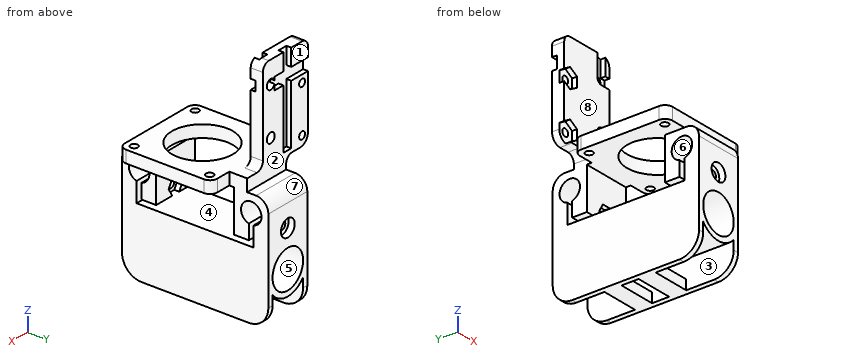
```python
from build123d import *

# Parameters (mm, degrees)
SKETCH_1_W                = 15.5
SKETCH_1_H                = 11.302783866
EXTRUDE_1_DEPTH           = 60
SKETCH_2_R                = 4.2
CUT_EXTRUDE_1_DEPTH       = 90
CUT_EXTRUDE_2_DEPTH       = 40
SKETCH_4_W                = 15.5
SKETCH_4_H                = 19.5
SKETCH_4_H_2              = 7
CUT_EXTRUDE_3_DEPTH       = 6
FILLET_1_R                = 5
FILLET_2_R                = 8
SKETCH_13_R               = 1.8
CUT_EXTRUDE_9_DEPTH       = 75
SKETCH_8_W                = 19.8
SKETCH_8_H                = 7.315078523
SKETCH_8_H_2              = 8
EXTRUDE_3_DEPTH           = 5
SKETCH_10_R               = 12.5
SKETCH_10_R_2             = 1.5
CUT_EXTRUDE_6_DEPTH       = 5
FILLET_4_R                = 3
CUT_EXTRUDE_10_DEPTH      = 34
CUT_EXTRUDE_10_DEPTH_BACK = 2
SKETCH_15_R               = 3.5
CUT_EXTRUDE_11_DEPTH      = 2.5
CUT_EXTRUDE_START         = -2.5
SKETCH_16_R               = 3.5
CUT_EXTRUDE_12_DEPTH      = 2.5
SKETCH_17_W               = 22.9
SKETCH_17_H               = 5
EXTRUDE_4_DEPTH           = 38
SKETCH_18_R               = 1.5
SKETCH_18_R_2             = 2
CUT_EXTRUDE_13_DEPTH      = 36.5
CUT_EXTRUDE_14_DEPTH      = 2
FILLET_5_R                = 3
SKETCH_20_W               = 4.5
SKETCH_20_H               = 5
SKETCH_20_W_2             = 4
SKETCH_20_W_3             = 8.5
SKETCH_20_H_2             = 6.981759249
SKETCH_20_H_3             = 24.431763341
CUT_EXTRUDE_15_DEPTH      = 2
FILLET_6_R                = 4
SKETCH_22_W               = 4
SKETCH_22_H               = 4
SKETCH_22_H_2             = 8.955168194
CUT_EXTRUDE_16_DEPTH      = 2


with BuildPart() as part:
    # Эскиз1 → Бобышка-Вытянуть1 (new body)
    with BuildSketch(Plane(origin=(0, 0, 0), x_dir=(1, 0, 0), z_dir=(0, 1, 0))):
        with BuildLine():
            Line((7.75, 0), (7.75, 6.160154219))
            ThreePointArc((7.75, 6.160154219), (0, 9.9), (-7.75, 6.160154219))
            Line((-7.75, 6.160154219), (-7.75, -3.2e-08))
            ThreePointArc((-7.75, -3.2e-08), (-1.6e-08, 7.75), (7.75, 0))
        make_face()
        with BuildLine():
            ThreePointArc((0, -9.9), (4.302584876, -8.916151826), (7.75, -6.160154219))
            Line((7.75, -6.160154219), (7.75, 0))
            ThreePointArc((7.75, 0), (1.6e-08, -7.75), (-7.75, -3.2e-08))
            Line((-7.75, -3.2e-08), (-7.75, -6.160154219))
            ThreePointArc((-7.75, -6.160154219), (-4.302584876, -8.916151826), (0, -9.9))
        make_face()
        with BuildLine():
            ThreePointArc((7.75, 6.160154219), (9.347058361, 3.262284476), (9.9, 0))
            Line((9.9, 0), (9.9, 18))
            Line((9.9, 18), (-9.9, 18))
            Line((-9.9, 18), (-9.9, 0))
            ThreePointArc((-9.9, 0), (-9.347058361, 3.262284476), (-7.75, 6.160154219))
            Line((-7.75, 6.160154219), (-7.75, 14))
            Line((-7.75, 14), (7.75, 14))
            Line((7.75, 14), (7.75, 6.160154219))
        make_face()
        with BuildLine():
            ThreePointArc((7.75, -6.160154219), (9.347058361, -3.262284476), (9.9, 0))
            ThreePointArc((9.9, 0), (9.347058361, 3.262284476), (7.75, 6.160154219))
            Line((7.75, 6.160154219), (7.75, 0))
            Line((7.75, 0), (7.75, -6.160154219))
        make_face()
        with BuildLine():
            Line((-7.75, -3.2e-08), (-7.75, 6.160154219))
            ThreePointArc((-7.75, 6.160154219), (-9.347058361, 3.262284476), (-9.9, 0))
            ThreePointArc((-9.9, 0), (-9.347058361, -3.262284476), (-7.75, -6.160154219))
            Line((-7.75, -6.160154219), (-7.75, -3.2e-08))
        make_face()
        with BuildLine():
            Line((9.9, -29), (9.9, 0))
            ThreePointArc((9.9, 0), (9.347058361, -3.262284476), (7.75, -6.160154219))
            Line((7.75, -6.160154219), (7.75, -9.9))
            Line((7.75, -9.9), (7.75, -11.85))
            Line((7.75, -11.85), (7.75, -23.152783866))
            Line((7.75, -23.152783866), (-7.75, -23.152783866))
            Line((-7.75, -23.152783866), (-7.75, -11.85))
            Line((-7.75, -11.85), (-7.75, -9.9))
            Line((-7.75, -9.9), (-7.75, -6.160154219))
            ThreePointArc((-7.75, -6.160154219), (-9.347058361, -3.262284476), (-9.9, 0))
            Line((-9.9, 0), (-9.9, -29))
            Line((-9.9, -29), (9.9, -29))
        make_face()
        with Locations((0, -17.501391933)):
            Rectangle(SKETCH_1_W, SKETCH_1_H)
        Polygon((7.75, -11.85), (7.75, -9.9), (0, -9.9), (-7.75, -9.9), (-7.75, -11.85), align=None)
        with BuildLine():
            Line((7.75, -9.9), (7.75, -6.160154219))
            ThreePointArc((7.75, -6.160154219), (4.302584876, -8.916151826), (0, -9.9))
            Line((0, -9.9), (7.75, -9.9))
        make_face()
        with BuildLine():
            Line((-7.75, -9.9), (0, -9.9))
            ThreePointArc((0, -9.9), (-4.302584876, -8.916151826), (-7.75, -6.160154219))
            Line((-7.75, -6.160154219), (-7.75, -9.9))
        make_face()
    extrude(amount=EXTRUDE_1_DEPTH)

    # Эскиз2 → Вырез-Вытянуть1 (cut)
    with BuildSketch(Plane(origin=(9.9, 0, 0), x_dir=(0, 0, -1), z_dir=(1, 0, 0))):
        with Locations((-22, 53)):
            Circle(SKETCH_2_R)
        with Locations((-22, 7)):
            Circle(SKETCH_2_R)
    extrude(amount=-CUT_EXTRUDE_1_DEPTH, mode=Mode.SUBTRACT)

    # Эскиз3 → Вырез-Вытянуть2 (cut)
    with BuildSketch(Plane(origin=(9.9, 0, 0), x_dir=(0, 0, -1), z_dir=(1, 0, 0))):
        Polygon((-29, 46), (-29, 14), (-11.85, 14), (-11.85, 8), (-22, 8), (-22, 6), (-9.85, 6), (-9.85, 54), (-22, 54), (-22, 52), (-11.85, 52), (-11.85, 46), align=None)
    extrude(amount=-CUT_EXTRUDE_2_DEPTH, mode=Mode.SUBTRACT)

    # Эскиз4 → Вырез-Вытянуть3 (cut)
    with BuildSketch(Plane(origin=(0, 0, -18), x_dir=(-1, 0, 0), z_dir=(0, 0, -1))):
        with Locations((0, 50.25)):
            Rectangle(SKETCH_4_W, SKETCH_4_H)
        with Locations((0, 30)):
            Rectangle(SKETCH_4_W, SKETCH_4_H_2)
        with Locations((0, 9.75)):
            Rectangle(SKETCH_4_W, SKETCH_4_H)
    extrude(amount=-CUT_EXTRUDE_3_DEPTH, mode=Mode.SUBTRACT)

    # Скругление1
    fillet_1_edges = [part.edges().sort_by_distance(p)[0] for p in [
        (0, 60, 29),
        (0, 0, 29),
    ]]
    fillet(fillet_1_edges, radius=FILLET_1_R)

    # Скругление2
    fillet_2_edges = [part.edges().sort_by_distance(p)[0] for p in [
        (-8.825, 60, -18),
        (-8.825, 0, -18),
        (8.825, 0, -18),
        (8.825, 60, -18),
    ]]
    fillet(fillet_2_edges, radius=FILLET_2_R)

    # Эскиз13 → Вырез-Вытянуть9 (cut)
    with BuildSketch(Plane.XZ):
        with Locations(Location((0, 14.920784389, 0), (0, 0, 270))):
            Circle(SKETCH_13_R)
    extrude(amount=-CUT_EXTRUDE_9_DEPTH, mode=Mode.SUBTRACT)

    # Эскиз8 → Бобышка-Вытянуть3 (add)
    with BuildSketch(Plane.XY.offset(29)):
        Polygon((-9.9, 44), (-19, 44), (-19, 6), (-9.9, 6), (-9.9, 14), (9.9, 14), (9.9, 6), (19, 6), (19, 44), (9.9, 44), align=None)
        with Locations((0, 47.657539262)):
            Rectangle(SKETCH_8_W, SKETCH_8_H)
        with Locations((0, 10)):
            Rectangle(SKETCH_8_W, SKETCH_8_H_2)
    extrude(amount=EXTRUDE_3_DEPTH)

    # Эскиз10 → Вырез-Вытянуть6 (cut)
    with BuildSketch(Plane.XY.offset(34)):
        with Locations((0, 25)):
            Circle(SKETCH_10_R)
        with Locations((-15.5, 9.5)):
            Circle(SKETCH_10_R_2)
        with Locations((-15.5, 40.5)):
            Circle(SKETCH_10_R_2)
        with Locations((15.5, 9.5)):
            Circle(SKETCH_10_R_2)
        with Locations((15.5, 40.5)):
            Circle(SKETCH_10_R_2)
    extrude(amount=-CUT_EXTRUDE_6_DEPTH, mode=Mode.SUBTRACT)

    # Скругление4
    fillet_4_edges = [part.edges().sort_by_distance(p)[0] for p in [
        (-19, 6, 31.5),
        (19, 6, 31.5),
        (19, 44, 31.5),
        (-19, 44, 31.5),
    ]]
    fillet(fillet_4_edges, radius=FILLET_4_R)

    # Эскиз14 → Вырез-Вытянуть10 (cut, two sides: drawn at the far end of the back side and taken through both)
    with BuildSketch(Plane(origin=(0, 14, 0), x_dir=(1, 0, 0), z_dir=(0, 1, 0)).offset(-CUT_EXTRUDE_10_DEPTH_BACK)):
        Polygon((-1.772918194, -17.991568778), (1.772918194, -17.991568778), (3.545836387, -14.920784389), (1.772918194, -11.85), (-1.772918194, -11.85), (-3.545836387, -14.920784389), align=None)
    extrude(amount=CUT_EXTRUDE_10_DEPTH + CUT_EXTRUDE_10_DEPTH_BACK, mode=Mode.SUBTRACT)

    # Эскиз15 → Вырез-Вытянуть11 (cut)
    with BuildSketch(Plane(origin=(0, 60, 0), x_dir=(1, 0, 0), z_dir=(0, 1, 0))):
        with Locations(Location((0, -14.920784389, 0), (0, 0, 270))):
            Circle(SKETCH_15_R)
    extrude(amount=-CUT_EXTRUDE_11_DEPTH, mode=Mode.SUBTRACT)

    # Эскиз16 → Вырез-Вытянуть12 (cut)
    with BuildSketch(Plane.XZ.offset(CUT_EXTRUDE_START)):
        with Locations(Location((0, 14.920784389, 0), (0, 0, 90))):
            Circle(SKETCH_16_R)
    extrude(amount=CUT_EXTRUDE_12_DEPTH, mode=Mode.SUBTRACT)

    # Эскиз17 → Бобышка-Вытянуть4 (add)
    with BuildSketch(Plane.XY.offset(34)):
        with Locations((-9.55, 48.815078523)):
            Rectangle(SKETCH_17_W, SKETCH_17_H)
    extrude(amount=EXTRUDE_4_DEPTH)

    # Эскиз18 → Вырез-Вытянуть13 (cut)
    with BuildSketch(Plane(origin=(0, 51.315078523, 0), x_dir=(1, 0, 0), z_dir=(0, 1, 0))):
        with Locations(Location((-18, -57, 0), (0, 0, 270))):
            Circle(SKETCH_18_R)
        with Locations(Location((-18, -38, 0), (0, 0, 270))):
            Circle(SKETCH_18_R)
        with Locations(Location((-2.1, -63.044831806, 0), (0, 0, 270))):
            Circle(SKETCH_18_R_2)
        with Locations(Location((-2.1, -43.673036669, 0), (0, 0, 270))):
            Circle(SKETCH_18_R_2)
    extrude(amount=-CUT_EXTRUDE_13_DEPTH, mode=Mode.SUBTRACT)

    # Эскиз19 → Вырез-Вытянуть14 (cut)
    with BuildSketch(Plane.XZ.offset(-46.315078523)):
        Polygon((-18, 61.041451884), (-21.5, 59.020725942), (-21.5, 54.979274058), (-18, 52.958548116), (-14.5, 54.979274058), (-14.5, 59.020725942), align=None)
        Polygon((-18, 42.041451884), (-21.5, 40.020725942), (-21.5, 35.979274058), (-18, 33.958548116), (-14.5, 35.979274058), (-14.5, 40.020725942), align=None)
    extrude(amount=-CUT_EXTRUDE_14_DEPTH, mode=Mode.SUBTRACT)

    # Скругление5
    fillet_5_edges = [part.edges().sort_by_distance(p)[0] for p in [
        (-9.9, 48.815078523, 34),
        (1.9, 48.815078523, 34),
        (1.9, 48.815078523, 72),
        (-21, 48.815078523, 72),
    ]]
    fillet(fillet_5_edges, radius=FILLET_5_R)

    # Эскиз20 → Вырез-Вытянуть15 (cut)
    with BuildSketch(Plane(origin=(0, 51.315078523, 0), x_dir=(1, 0, 0), z_dir=(0, 1, 0))):
        with Locations((-6.25, -62.518240751)):
            Rectangle(SKETCH_20_W, SKETCH_20_H)
        with Locations((-10.5, -62.518240751)):
            Rectangle(SKETCH_20_W_2, SKETCH_20_H)
        with Locations((-16.75, -62.518240751)):
            Rectangle(SKETCH_20_W_3, SKETCH_20_H)
        with Locations((-10.5, -68.509120376)):
            Rectangle(SKETCH_20_W_2, SKETCH_20_H_2)
        with Locations((-10.5, -47.80235908)):
            Rectangle(SKETCH_20_W_2, SKETCH_20_H_3)
    extrude(amount=-CUT_EXTRUDE_15_DEPTH, mode=Mode.SUBTRACT)

    # Скругление6
    # the kernel refuses this fillet: 4 mm, written as the material it takes off along each edge
    with BuildSketch(Plane(origin=(-21, 61.315078523, 34), x_dir=(1, 0, 0), z_dir=(0, -1, 0))) as fillet_6_piece_1:
        with BuildLine():
            CenterArc((FILLET_6_R, FILLET_6_R), FILLET_6_R, 180, 90)
            Line((0, FILLET_6_R), (0, 0))
            Line((0, 0), (FILLET_6_R, 0))
        make_face()
    extrude(amount=25, mode=Mode.SUBTRACT)

    # Эскиз22 → Вырез-Вытянуть16 (cut)
    with BuildSketch(Plane.XZ.offset(-46.315078523)):
        with Locations((-0.1, 63.044831806)):
            Rectangle(SKETCH_22_W, SKETCH_22_H)
        with Locations((-2.1, 67.522415903)):
            Rectangle(SKETCH_22_W, SKETCH_22_H_2)
    extrude(amount=-CUT_EXTRUDE_16_DEPTH, mode=Mode.SUBTRACT)


solid = part.part
```
Input: part model. Units: mm. Frame: model coordinates. Face numbers are marked on the shaded views. A direction names the side the tool comes from. Coordinates: 2 decimals unless noted, no trailing zeros. Write each loop counter-clockwise with the first axis right and the second up, starting at its lowest first coordinate (ties: lowest second). Pieces come first, ordered by that corner, then holes. Notation, with made-up numbers: (37, 57.25) -> (49, 57.25) arc R24 cw to (49, 73.25) -> close; hole circle Ø9 at (-22, 68). An arc over 180 degrees is marked (long way). Answer as a JSON object with one key per item and string values.
1. Section A-A on y = 25. Return the cut outline in (x, z).
Result set:
{"outline": "(-19, 29) -> (-12.5, 29) -> (-12.5, 34) -> (-19, 34) -> close; (-9.9, -18) -> (9.9, -18) -> (9.9, 9.85) -> (-9.9, 9.85) -> close; (12.5, 29) -> (19, 29) -> (19, 34) -> (12.5, 34) -> close; hole (-7.75, -14) -> (7.75, -14) -> (7.75, -6.16) arc R9.9 cw to (-7.75, -6.16) -> close; hole circle Ø15.5 at (0, 0)"}
2. Material intervals for line 1 (Y direction, x = 0.25, z = 22); line 2 (X direction, y = 50, z = 57); line 3 (X direction, y = 25, z = 33.05), sorted ascending. Write a range as from..to.
Result set:
{"line 1": "y = 0..2.8, 11.2..14, 46..48.8, 57.2..60", "line 2": "x = -21..-19.5, -16.5..-12.5, -8.5..1.9", "line 3": "x = -19..-12.5, 12.5..19"}
3. Access query for the marked faces 1, 2, 3, 4 and 5. Directions: +Z, -Z, +X, -X, +Y, -Y. A direction counts if a zero-diameter tool reaches every point of the face in a straight line with its end or side. Return the directions, or none.
Result set:
{"face 1": "+Z, -Z, +X, -X, +Y", "face 2": "+Z, +X, -X, +Y", "face 3": "none", "face 4": "+X, -X", "face 5": "+Y, -Y"}
4. Section D-D on z = 44. Return the cut outline in (x, y), then the cut area to 3 significant figures.
Result set:
{"outline": "(-21, 46.32) -> (-4.07, 46.32) -> (-4.07, 51.32) -> (-8.5, 51.32) -> (-8.5, 49.32) -> (-12.5, 49.32) -> (-12.5, 51.32) -> (-21, 51.32) -> close; (-0.13, 46.32) -> (1.9, 46.32) -> (1.9, 51.32) -> (-0.13, 51.32) -> close", "area": "86.8 mm2"}
5. First-contact query: P1, Ø0.6, axis at x = -6.5, y = 51, coming from the -Z side; P2, Ø3, axis at x = 9.5, z = 34.5, coming from the +Y side; P3, Ø0.6, axis at x = -11, y = 50.5, coming from the +Z side. Flat tips, straight axial feed; report the tip coordinate or a pass-through.
Result set:
{"P1": "stops at z = -7.72", "P2": "stops at y = 51.32", "P3": "stops at z = 35.59"}
6. Mould query, pull axis Z, two halves, no side actions, for the marked faces 6, 7 and 8. Classes: released by +Z, released by -Z, zero draft, split by the parting line, or undercut.
Result set:
{"face 6": "undercut", "face 7": "released by +Z", "face 8": "zero draft"}
7. Section B-B on z = 22. Return the cut outline in (x, y), then the cut area to 3 significant figures.
Result set:
{"outline": "(-9.9, 0) -> (9.9, 0) -> (9.9, 2.8) -> (-9.9, 2.8) -> close; (-9.9, 11.2) -> (9.9, 11.2) -> (9.9, 14) -> (-9.9, 14) -> close; (-9.9, 46) -> (9.9, 46) -> (9.9, 48.8) -> (-9.9, 48.8) -> close; (-9.9, 57.2) -> (9.9, 57.2) -> (9.9, 60) -> (-9.9, 60) -> close", "area": "222 mm2"}
8. Section C-C on y = 53. Return the cut outline in (x, z).
Result set:
{"outline": "(-9.9, -17.94) -> (-7.75, -17.94) -> (-7.75, -6.16) arc R9.9 ccw to (7.75, -6.16) -> (7.75, -17.94) -> (9.9, -17.94) -> (9.9, 9.85) -> (-9.9, 9.85) -> close; (-9.9, 26.2) -> (9.9, 26.2) -> (9.9, 29) -> (-9.9, 29) -> close; hole circle Ø15.5 at (0, 0)"}
